For this review, take the finished solid that the model builds, in its own axes (mm). Face numbers are marked on the shaded views. A direction names the side the tool comes from. Give positions to 0.01 mm unless a question says otherwise; leave off trailing zeros. Order: outer loops, then holes, each group sorted by start corner. A loop starts at its lowest first (then second) coordinate and runs counter-clockwise, first axis right, second up. Notation, with made-up numbers: (-25.75, -13) -> (2.25, -13) arc R10 cw to (2.25, -1) -> close; hole circle Ø6 at (47, 20.25). An arc over 180 degrees is marked (long way). Use CSV: the item, a comma, the result in double quotes. Start each with the question number.
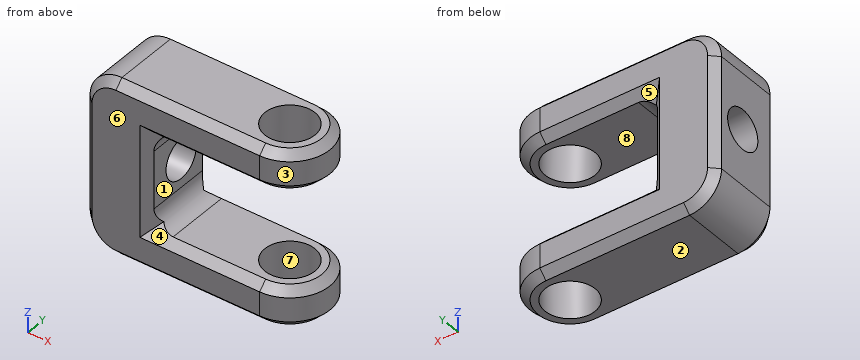
```python
from build123d import *

# Parameters (mm, degrees)
SKETCH1_R           = 4.9609375
BOSS_EXTRUDE1_DEPTH = 34.925
SKETCH2_W           = 30.1625
SKETCH2_H           = 19.05
CUT_EXTRUDE1_DEPTH  = 16.875
SKETCH3_R           = 3.96875
CUT_EXTRUDE2_DEPTH  = 43.8625
FILLET1_R           = 6.35
CHAMFER1_SIZE       = 1.5875
FILLET2_R           = 3.81


with BuildPart() as part:
    # Sketch1 → Boss-Extrude1 (new body)
    with BuildSketch(Plane.XY):
        with BuildLine():
            Line((0, 0), (34.925, 0))
            ThreePointArc((34.925, 0), (42.8625, 7.9375), (34.925, 15.875))
            Line((34.925, 15.875), (0, 15.875))
            Line((0, 15.875), (0, 0))
        make_face()
        with Locations((34.925, 7.9375)):
            Circle(SKETCH1_R, mode=Mode.SUBTRACT)
    extrude(amount=BOSS_EXTRUDE1_DEPTH)

    # Sketch2 → Cut-Extrude1 (cut, through all)
    with BuildSketch(Plane(origin=(0, 15.875, 0), x_dir=(1, 0, 0), z_dir=(0, 1, 0))):
        with Locations((27.78125, -17.4625)):
            Rectangle(SKETCH2_W, SKETCH2_H)
    extrude(amount=-CUT_EXTRUDE1_DEPTH, mode=Mode.SUBTRACT)

    # Sketch3 → Cut-Extrude2 (cut, through all)
    with BuildSketch(Plane.ZY):
        with Locations((17.4625, 8.73125)):
            Circle(SKETCH3_R)
    extrude(amount=-CUT_EXTRUDE2_DEPTH, mode=Mode.SUBTRACT)

    # Fillet1
    fillet1_edges = [part.edges().sort_by_distance(p)[0] for p in [
        (0, 7.9375, 34.925),
        (0, 7.9375, 0),
    ]]
    fillet(fillet1_edges, radius=FILLET1_R)

    # Chamfer1
    chamfer1_edges = [part.edges().sort_by_distance(p)[0] for p in [
        (42.8625, 7.9375, 34.925),
        (20.6375, 15.875, 34.925),
        (23.8125, 15.875, 26.9875),
        (23.8125, 15.875, 7.9375),
        (12.7, 15.875, 17.4625),
        (42.8625, 7.9375, 7.9375),
        (23.8125, 0, 7.9375),
        (42.8625, 7.9375, 26.9875),
        (23.8125, 0, 26.9875),
        (12.7, 0, 17.4625),
        (20.6375, 15.875, 0),
        (0, 0, 17.4625),
        (0, 15.875, 17.4625),
        (42.8625, 7.9375, 0),
        (20.6375, 0, 34.925),
        (20.6375, 0, 0),
        (1.859871939, 0, 33.065128061),
        (1.859871939, 0, 1.859871939),
        (1.859871939, 15.875, 33.065128061),
        (1.859871939, 15.875, 1.859871939),
    ]]
    chamfer(chamfer1_edges, length=CHAMFER1_SIZE)

    # Fillet2
    fillet2_edges = [part.edges().sort_by_distance(p)[0] for p in [
        (12.7, 7.9375, 26.9875),
        (12.7, 7.9375, 7.9375),
    ]]
    fillet(fillet2_edges, radius=FILLET2_R)


solid = part.part
```
1. To check wall thickness, follow L1, parallel to Z at x = 25, y = 5.25 (1 decimal); L2, parallel to X at y = 11, z = 21.5; L3, parallel to X at y = 5.5, z = 28.5. State the ranges of each line that lie inside material, in increasing order. Write a range as [from, to].
2. Clearance check with flat-ended pins moving along their axes: P1, Ø4, axis at y = 2, z = 18, coming from the +X side; P2, Ø5, axis at x = 24, z = 26, coming from the -Y side (3 decimals). State where each tip first meets the part, or that it passes through.
3. For the marked faces 4, 5, 6, 7 and 8, list the 3-axis set-ups (+Z, -Z, +X, -X, +Y, -Y) from which the entire face can be reached by the end or side of a thin tool; tool diameter is ignored.
4. Draft analysis for pull direction Z (two halves, no side actions). For the marked faces 1, 2 and 3, state which applies: +Z half, -Z half, draft (parallel to the pull), parting line (faces both ways), or undercut.
5. Consider section C-C (z = 11). State the section outline as (x, y) points (1 decimal), plus the area to 3 significant figures.
6. Consider section B-B (x = 31). State how many separate pieces and enclosed holes the cut face has, plus the area to 3 significant figures.
Answer list:
1,L1,"[0, 7.9], [27, 34.9]"
1,L2,"[0, 12.7]"
1,L3,"[0, 30.6], [39.25, 42.4]"
2,P1,"x = 12.7"
2,P2,"y = 0.075"
3,face 4,"+X, -Y"
3,face 5,"+X, +Y"
3,face 6,"+Z, -Z, +X, -X, -Y"
3,face 7,"+Z, -Z"
3,face 8,"+X, +Y, -Y"
4,face 1,"undercut"
4,face 2,"-Z half"
4,face 3,"draft"
5,outline,"(0, 1.6) -> (1.6, 0) -> (11.1, 0) -> (12.8, 1.7) -> (12.8, 14.2) -> (11.1, 15.9) -> (1.6, 15.9) -> (0, 14.3) -> close"
5,area,"198 mm2"
6,separate pieces,"4"
6,enclosed holes,"0"
6,area,"146 mm2"
